```python
from build123d import *

# Parameters (mm, degrees)
SKETCH1_W           = 19.05
SKETCH1_H           = 19.05
SKETCH1_R           = 0.79375
BOSS_EXTRUDE1_DEPTH = 3.175
FILLET2_R           = 0.635


with BuildPart() as part:
    # Sketch1 → Boss-Extrude1 (new body)
    with BuildSketch(Plane.XY):
        Rectangle(SKETCH1_W, SKETCH1_H)
        with Locations((-4.826, -6.477)):
            Circle(SKETCH1_R, mode=Mode.SUBTRACT)
        with Locations((4.826, -6.477)):
            Circle(SKETCH1_R, mode=Mode.SUBTRACT)
        with Locations(Location((4.826, 6.477, 0), (0, 0, 180))):
            Circle(SKETCH1_R, mode=Mode.SUBTRACT)
        with Locations(Location((-4.826, 6.477, 0), (0, 0, 180))):
            Circle(SKETCH1_R, mode=Mode.SUBTRACT)
    extrude(amount=BOSS_EXTRUDE1_DEPTH)

    # Fillet2
    fillet2_edges = [part.edges().sort_by_distance(p)[0] for p in [
        (0, -9.525, 3.175),
        (9.525, 0, 3.175),
        (0, 9.525, 3.175),
        (9.525, 0, 0),
        (0, -9.525, 0),
        (-9.525, 0, 0),
        (0, 9.525, 0),
        (9.525, 9.525, 1.5875),
        (9.525, -9.525, 1.5875),
        (-9.525, -9.525, 1.5875),
        (-9.525, 9.525, 1.5875),
        (-9.525, 0, 3.175),
    ]]
    fillet(fillet2_edges, radius=FILLET2_R)


solid = part.part
```
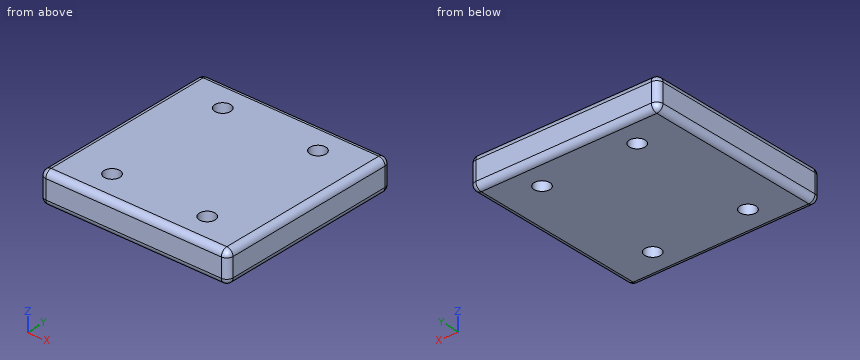
CAD build for the part. Positions are in the model's coordinates, mm. Give positions to 0.01 mm unless a question says otherwise; leave off trailing zeros. Order: outer loops, then holes, each group sorted by start corner. A loop starts at its lowest first (then second) coordinate and runs counter-clockwise, first axis right, second up.
(1) Drill centre lines: L1, parallel to X at y = 7, z = 3; L2, parallel to Y at x = 5.25, z = 0.35; L3, parallel to X at y = -3.75, z = 0.55. Where is each one in solid material? Low to high.
(2) Saw through at A-A, the plane x = -4.75. Give the cut face in (y, z) (3 decimals).
(3) Saw through at C-C, the plane x = 4.5. Give the cut face in (y, z) (3 decimals).
(4) Saw through at B-B, the plane z = 1.5. Give the cut face in (x, y) (1 decimal), then the cut area to 3 significant figures.
Results found:
1. L1: x = -9.33 to -5.42, -4.23 to 4.23, 5.42 to 9.33
1. L2: y = -9.46 to -7.15, -5.81 to 5.81, 7.15 to 9.46
1. L3: x = -9.52 to 9.52
2. outline: (-9.525, 0.635) arc R0.635 ccw to (-8.89, 0) - (-7.267, 0) - (-7.267, 3.175) - (-8.89, 3.175) arc R0.635 ccw to (-9.525, 2.54) - close; (-5.687, 0) - (5.687, 0) - (5.687, 3.175) - (-5.687, 3.175) - close; (7.267, 0) - (8.89, 0) arc R0.635 ccw to (9.525, 0.635) - (9.525, 2.54) arc R0.635 ccw to (8.89, 3.175) - (7.267, 3.175) - close
3. outline: (-9.525, 0.635) arc R0.635 ccw to (-8.89, 0) - (-7.201, 0) - (-7.201, 3.175) - (-8.89, 3.175) arc R0.635 ccw to (-9.525, 2.54) - close; (-5.753, 0) - (5.753, 0) - (5.753, 3.175) - (-5.753, 3.175) - close; (7.201, 0) - (8.89, 0) arc R0.635 ccw to (9.525, 0.635) - (9.525, 2.54) arc R0.635 ccw to (8.89, 3.175) - (7.201, 3.175) - close
4. outline: (-9.5, -8.9) arc R0.6 ccw to (-8.9, -9.5) - (8.9, -9.5) arc R0.6 ccw to (9.5, -8.9) - (9.5, 8.9) arc R0.6 ccw to (8.9, 9.5) - (-8.9, 9.5) arc R0.6 ccw to (-9.5, 8.9) - close; hole circle Ø1.6 at (-4.8, -6.5); hole circle Ø1.6 at (-4.8, 6.5); hole circle Ø1.6 at (4.8, -6.5); hole circle Ø1.6 at (4.8, 6.5)
4. area: 355 mm2
